from build123d import *

# Parameters (mm, degrees)
EXTRUDE008_DEPTH                          = 7
EXTRUDE008_ONTO_SKETCH008_ROLL_ANGLE      = 90
EXTRUDE008_ONTO_SKETCH008_PITCH_ANGLE     = -30
EXTRUDE008_ONTO_SKETCH008_PLACEMENT_ANGLE = -90
SKETCH004_W                               = 87.248978
SKETCH004_H                               = 34.299007
EXTRUDE004_DEPTH                          = 10
EXTRUDE006_DEPTH                          = 7
EXTRUDE006_ONTO_SKETCH_ROLL_ANGLE         = 90
EXTRUDE006_ONTO_SKETCH_PITCH_ANGLE        = -30
EXTRUDE006_ONTO_SKETCH_PLACEMENT_ANGLE    = -90
SKETCH007_W                               = 88
SKETCH007_H                               = 88
SKETCH007_R                               = 38
EXTRUDE007_DEPTH                          = 7
EXTRUDE007_PLACEMENT_ANGLE                = 30
SKETCH005_W                               = 88
SKETCH005_H                               = 13
EXTRUDE005_DEPTH                          = 64


with BuildPart() as extrude008:
    # Sketch008 as drawn → Extrude008 (new)
    with BuildSketch(Plane.XY):
        Polygon((-123.305188, 6.070855), (-123.344503, -1.169558), (-100.406639, -23.66512), (-15.520081, -91.56636), (-9.4672, -97.367993), (-1.018409, -90.281281), (-3.036737, -87.875028), (-34.868234, 6.09489), align=None)
    extrude(amount=EXTRUDE008_DEPTH)


with BuildPart() as extrude008_1:
    # Extrude008 onto Sketch008 roll: moved
    add(extrude008.part.rotate(Axis((0, 0, 0), (1, 0, 0)), EXTRUDE008_ONTO_SKETCH008_ROLL_ANGLE))


with BuildPart() as extrude008_2:
    # Extrude008 onto Sketch008 pitch: moved
    add(extrude008_1.part.rotate(Axis((0, 0, 0), (0, 1, 0)), EXTRUDE008_ONTO_SKETCH008_PITCH_ANGLE))


with BuildPart() as extrude008_3:
    # Extrude008 onto Sketch008 placement: moved
    add(extrude008_2.part.moved(Location((42.577726, 14, 39))).rotate(Axis((42.577726, 14, 39), (0, 0, 1)), EXTRUDE008_ONTO_SKETCH008_PLACEMENT_ANGLE))


with BuildPart() as extrude008_4:
    # Extrude008 placement: moved
    add(extrude008_3.part.moved(Location((7, 0, 0))))


with BuildPart() as extrude004:
    # Sketch004 → Extrude004 (new body)
    with BuildSketch(Plane.XY):
        with Locations((83.604523, 30.688192)):
            Rectangle(SKETCH004_W, SKETCH004_H)
    extrude(amount=EXTRUDE004_DEPTH)


with BuildPart() as extrude004_1:
    # Extrude004 placement: moved
    add(extrude004.part.moved(Location((3, 0, 9))))


with BuildPart() as extrude006:
    # Sketch as drawn → Extrude006 (new)
    with BuildSketch(Plane.XY):
        Polygon((-123.305188, 6.070855), (-123.344503, -1.169558), (-100.406639, -23.66512), (-15.520081, -91.56636), (-9.4672, -97.367993), (-1.018409, -90.281281), (-3.036737, -87.875028), (-34.868234, 6.09489), align=None)
    extrude(amount=EXTRUDE006_DEPTH)


with BuildPart() as extrude006_1:
    # Extrude006 onto Sketch roll: moved
    add(extrude006.part.rotate(Axis((0, 0, 0), (1, 0, 0)), EXTRUDE006_ONTO_SKETCH_ROLL_ANGLE))


with BuildPart() as extrude006_2:
    # Extrude006 onto Sketch pitch: moved
    add(extrude006_1.part.rotate(Axis((0, 0, 0), (0, 1, 0)), EXTRUDE006_ONTO_SKETCH_PITCH_ANGLE))


with BuildPart() as extrude006_3:
    # Extrude006 onto Sketch placement: moved
    add(extrude006_2.part.moved(Location((42.577726, 14, 39))).rotate(Axis((42.577726, 14, 39), (0, 0, 1)), EXTRUDE006_ONTO_SKETCH_PLACEMENT_ANGLE))


with BuildPart() as extrude006_4:
    # Extrude006 placement: moved
    add(extrude006_3.part.moved(Location((88, 0, 0))))


with BuildPart() as extrude007:
    # Sketch007 → Extrude007 (new body)
    with BuildSketch(Plane.XY):
        with Locations((83.189821, 78.875904)):
            Rectangle(SKETCH007_W, SKETCH007_H)
        with Locations((83.189821, 78.875904)):
            Circle(SKETCH007_R, mode=Mode.SUBTRACT)
    extrude(amount=EXTRUDE007_DEPTH)


with BuildPart() as extrude007_1:
    # Extrude007 placement: moved
    add(extrude007.part.moved(Location((3, 14, 39))).rotate(Axis((3, 14, 39), (-1, 0, 0)), EXTRUDE007_PLACEMENT_ANGLE))


with BuildPart() as suporte2:
    # Sketch005 → Extrude005 (new body)
    with BuildSketch(Plane.XY):
        with Locations((83.577726, 41.368692)):
            Rectangle(SKETCH005_W, SKETCH005_H)
    extrude(amount=EXTRUDE005_DEPTH)


with BuildPart() as suporte2_1:
    # Extrude005 placement: moved
    add(suporte2.part.moved(Location((3, 0, 19))))

    # Fusion: union Extrude008, Extrude004, Extrude006, Extrude007
    add(extrude008_4.part)
    add(extrude004_1.part)
    add(extrude006_4.part)
    add(extrude007_1.part)


solid = suporte2_1.part
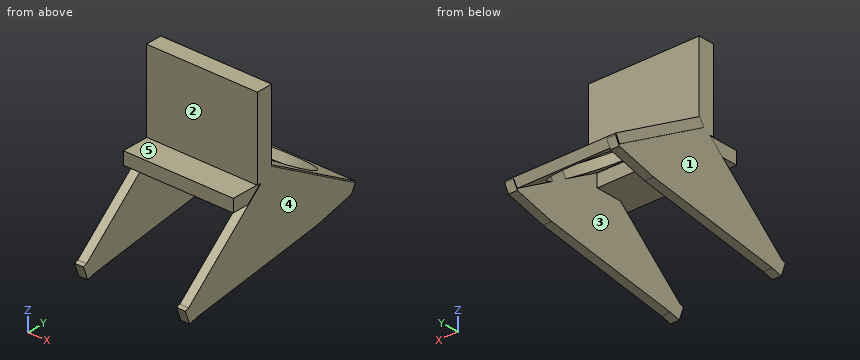
CAD build for the part. Positions are in the model's coordinates, mm. Face numbers are marked on the shaded views. A direction names the side the tool comes from. Coordinates: 2 decimals unless noted, no trailing zeros. Loops run counter-clockwise (first coordinate to the right, second up) from the corner with the lowest first, then second, coordinate; pieces in that order, holes last. Notation, with made-up numbers: (-1.5, -6) -> (23.5, -6) arc R13 cw to (23.5, -2) -> close; hole circle Ø8 at (2, 50). An arc over 180 degrees is marked (long way). One line per item, written item: value.
1. Slice it at C-C on z = 72. Write the cut outline in (x, y), and give its area (3 significant figures).
Answers:
outline: (42.58, 34.87) -> (130.58, 34.87) -> (130.58, 47.87) -> (42.58, 47.87) -> close
area: 1,140 mm^2
2. Slice it at B-B on y = 4.5. Write the cut outline in (x, z), and give its area (3 significant figures).
Answers:
outline: (42.58, -44.58) -> (49.58, -44.58) -> (49.58, -10.69) -> (42.58, -10.69) -> close; (123.58, -44.58) -> (130.58, -44.58) -> (130.58, -10.69) -> (123.58, -10.69) -> close
area: 474 mm^2
3. Drill centre lines: line 1 (X direction, y = 91, z = -8); line 2 (X direction, y = 45.5, z = 46); line 3 (Z direction, x = 55, y = 46). Where is each one in solid material? Low to high. Write a range as [from, to].
Answers:
line 1: x = [42.58, 49.58], [123.58, 130.58]
line 2: x = [42.58, 130.58]
line 3: z = [9, 83]
4. Flat gauge pins, fed straight in: P1, Ø19, axis at x = 98.5, z = 56, coming from the -Y side; P2, Ø21, axis at y = 64, z = -23, coming from the -X side; P3, Ø10.5, axis at x = 105, y = 37.5, coming from the -Z side; P4, Ø22.5, axis at y = 92.5, z = 11, coming from the +X side. Where does each tip first touch, or does it go through?
Answers:
P1: stops at y = 34.87
P2: stops at x = 42.58
P3: stops at z = 9
P4: stops at x = 130.58
5. Pull direction X, two halves, no side cores. Call the marked faces 1, 2 and 3: pulls with the +X half, pulls with the -X half, needs draft (parallel to the pull), parting line crosses it, or undercut.
Answers:
face 1: pulls with the -X half
face 2: needs draft
face 3: undercut
6. Which spindle directions (+Z, -Z, +X, -X, +Y, -Y) get a long thin tool onto all of the face, cutting with end or side? Do the marked faces 4 and 5. Say none if no direction does.
Answers:
face 4: +Z, -Z, +X, +Y, -Y
face 5: +Z, +X, -X, -Y
